from build123d import *

# Parameters (mm, degrees)
SKETCH_1_R      = 1.5
SKETCH_1_R_2    = 2
EXTRUDE_1_DEPTH = 6


with BuildPart() as part:
    # Sketch 1 → Extrude 1 (new body)
    with BuildSketch(Plane.XY):
        Polygon((-57.5, 129.437494331), (57.5, 129.437494331), (57.5, 99.437494331), (41.992637301, 99.437494331), (41.992637301, -45.562505669), (57.5, -45.562505669), (57.5, -80.562505669), (-57.5, -80.562505669), (-57.5, -45.562505669), (-41.992637301, -45.562505669), (-41.992637301, 99.437494331), (-57.5, 99.437494331), align=None)
        with Locations((-51.105648031, 119.710621144)):
            Circle(SKETCH_1_R, mode=Mode.SUBTRACT)
        with Locations((51.105648031, 119.710621144)):
            Circle(SKETCH_1_R, mode=Mode.SUBTRACT)
        with Locations((-47.5, -53.062505669)):
            Circle(SKETCH_1_R, mode=Mode.SUBTRACT)
        with Locations((47.5, -53.062505669)):
            Circle(SKETCH_1_R, mode=Mode.SUBTRACT)
        with Locations((-25, 96.939287159)):
            Circle(SKETCH_1_R_2, mode=Mode.SUBTRACT)
        with Locations((25, 96.939287159)):
            Circle(SKETCH_1_R_2, mode=Mode.SUBTRACT)
        with Locations((-25, -48.062505669)):
            Circle(SKETCH_1_R_2, mode=Mode.SUBTRACT)
        with Locations((25, -48.062505669)):
            Circle(SKETCH_1_R_2, mode=Mode.SUBTRACT)
        with Locations((7, 36.937494331)):
            Circle(SKETCH_1_R, mode=Mode.SUBTRACT)
    extrude(amount=EXTRUDE_1_DEPTH)


solid = part.part
The model under review builds one solid part; all positions refer to its coordinate system, in mm. A direction names the side the tool comes from. Round coordinates to 2 decimals unless told otherwise and drop trailing zeros. Order: outer loops, then holes, each group sorted by start corner. A loop starts at its lowest first (then second) coordinate and runs counter-clockwise, first axis right, second up. Notation, with made-up numbers: (14.5, 76.5) - (69.5, 76.5) arc R26 cw to (69.5, 90.5) - close; hole circle Ø5 at (9.25, 32.25). An arc over 180 degrees is marked (long way). Use one line per item in the form item = value.
Q1. Mouldability with a two-part tool opening along X and no side actions: class faces 4 (the flat face through (57.5, -63, 3)), 5 (the cylindrical face through (-25.434, -50.015, 2.958)), 6 (the flat face through (50, 99.437, 3)) as pulls with the +X half, pulls with the -X half, needs draft (parallel to the pull), parting line crosses it, or undercut.
Response values:
face_4 = pulls with the +X half
face_5 = undercut
face_6 = needs draft
Q2. Tool access review of faces 1 (the flat face through (41.993, 28, 3)), 2 (the flat face through (-50, 99.437, 3)), 3 (the flat face through (-57.5, -63, 3)): name each direction out of +Z, -Z, +X, -X, +Y, -Y from which nothing blocks a thin tool from reaching the whole face with its end or side.
Response values:
face_1 = +Z, -Z, +X
face_2 = +Z, -Z, -X
face_3 = +Z, -Z, -X, +Y, -Y
Q3. Add section A-A on x = -25. Give the boundary of the cut face in (y, z).
Response values:
outline = (-80.56, 0) - (-50.06, 0) - (-50.06, 6) - (-80.56, 6) - close; (-46.06, 0) - (94.94, 0) - (94.94, 6) - (-46.06, 6) - close; (98.94, 0) - (129.44, 0) - (129.44, 6) - (98.94, 6) - close
Q4. Add section B-B on z = 3.75. Give the number of separate pieces and of enclosed holes in the cut face, then the cut area to 3 significant figures.
Response values:
separate_pieces = 1
enclosed_holes = 9
area = 19,600 mm^2
Q5. Add section C-C on y = -16. Give the boundary of the cut face in (x, z), then the cut area to 3 significant figures.
Response values:
outline = (-41.99, 0) - (41.99, 0) - (41.99, 6) - (-41.99, 6) - close
area = 504 mm^2
Q6. Clearance check with flat-ended pins moving along their axes: P1, Ø3.5, axis at x = -25, y = -48.06, coming from the -Z side; P2, Ø3, axis at y = -18.5, z = 5, coming from the -X side; P3, Ø1.5, axis at y = -23, z = 5, coming from the +X side. State where each tip first meets the part, or that it passes through.
Response values:
P1 = through
P2 = -41.99
P3 = 41.99
Q7. To check wall thickness, follow line 1 (Y direction, x = -25, z = 4.55); line 2 (Y direction, x = -43, z = 0.9); line 3 (Y direction, x = -50, z = 3.3). State the ranges of each line that lie inside material, in increasing order.
Response values:
line_1 = -80.56 to -50.06, -46.06 to 94.94, 98.94 to 129.44
line_2 = -80.56 to -45.56, 99.44 to 129.44
line_3 = -80.56 to -45.56, 99.44 to 118.7, 120.72 to 129.44
